The listing builds one solid part. Answer for the finished solid, in the listing's coordinates (mm). Face numbers are marked on the shaded views. A direction names the side the tool comes from. Round coordinates to 2 decimals unless told otherwise and drop trailing zeros. Order: outer loops, then holes, each group sorted by start corner. A loop starts at its lowest first (then second) coordinate and runs counter-clockwise, first axis right, second up. Notation, with made-up numbers: (-30, -8.5) - (-5, -8.5) arc R23 ccw to (-5, 13.5) - close; hole circle Ø2 at (28.25, 19.5). An arc over 180 degrees is marked (long way). One line per item, written item: value. Start each with the question number.
1. Section A-A, the plane z = 15.5 is taken. Give the vertices of the cut face in (x, y), then the cut area to 3 significant figures.
2. Flat-ended cylindrical pins translate along their axes: P1, Ø1, axis at x = -4, z = 14.5, coming from the +Y side; P2, Ø2, axis at x = -13, y = -5.5, coming from the -Z side; P3, Ø6, axis at x = -9.5, z = 15.5, coming from the -Y side; P4, Ø3.5, axis at y = -4, z = -7, coming from the +X side. Find the tip coordinate at first contact, or state that the pin passes through.
3. Straight lines are drawn through the part: line 1 (X direction, y = -5.75, z = 34.5); line 2 (X direction, y = -6.75, z = 40.5); line 3 (Z direction, x = -10, y = -0.55). For each, find the intervals that lie inside material, in ascending order.
4. Section C-C, the plane x = -1.5 is taken. Give the vertices of the cut face in (y, z), then the cut area to 4 significant figures.
5. Section D-D, the plane z = 8 is taken. Give the vertices of the cut face in (x, y).
6. Section B-B, the plane y = -10.5 is taken. Give the vertices of the cut face in (x, z), then the cut area to 4 significant figures.
7. A tool of negligible diameter and unlimited length cuts with its end or side. For the marked faces 1, 2, 3 and 4, from which of +Z, -Z, +X, -X, +Y, -Y can it reach the whole face along a straight path? Write none if from no direction.
from build123d import *

# Parameters (mm, degrees)
F0_W      = 8
F0_H      = 31
F1_DEPTH  = 20
F3_DEPTH  = 6.4
F4_R      = 2
F5_DEPTH  = 1.601
F9_W      = 4.8
F9_H      = 18
F10_DEPTH = 30
F12_DEPTH = 3
F13_R     = 2
F14_DEPTH = 1.801
F15_SIZE  = 0.5
F16_SIZE2 = 2
F16_SIZE  = 0.5
F17_SIZE  = 1


with BuildPart() as f1:
    # F0 (on Right) → F1 (new body)
    with BuildSketch(Plane.YZ):
        with Locations((-4, 15.5)):
            Rectangle(F0_W, F0_H)
    extrude(amount=-F1_DEPTH)

    # F2 (on face) → F3 (cut)
    with BuildSketch(Plane.XZ.offset(8)):
        Polygon((-6.45, 13.4504065444), (-6.45, 17.5495934556), (-10, 19.5991869112), (-13.55, 17.5495934556), (-13.55, 13.4504065444), (-10, 11.4008130888), align=None)
    extrude(amount=-F3_DEPTH, mode=Mode.SUBTRACT)

    # F4 (on face) → F5 (cut, through all)
    with BuildSketch(Plane.XZ.offset(1.6)):
        with Locations((-10, 15.5)):
            Circle(F4_R)
    extrude(amount=-F5_DEPTH, mode=Mode.SUBTRACT)

    # F9 (on 3pt) → F10 (join, symmetric)
    with BuildSketch(Plane.XY.offset(15.5)):
        with Locations((2.4, -4)):
            Rectangle(F9_W, F9_H)
    extrude(amount=F10_DEPTH, both=True)

    # F11 (on face) → F12 (cut)
    with BuildSketch(Plane(origin=(0, 0, 0), x_dir=(0, -1, 0), z_dir=(-1, 0, 0))):
        Polygon((6.0495934556, 41.55), (1.9504065444, 41.55), (-0.0991869112, 38), (1.9504065444, 34.45), (6.0495934556, 34.45), (8.0991869112, 38), align=None)
        Polygon((6.0495934556, -3.45), (1.9504065444, -3.45), (-0.0991869112, -7), (1.9504065444, -10.55), (6.0495934556, -10.55), (8.0991869112, -7), align=None)
    extrude(amount=-F12_DEPTH, mode=Mode.SUBTRACT)

    # F13 (on face) → F14 (cut, through all)
    with BuildSketch(Plane(origin=(3, 0, 0), x_dir=(0, -1, 0), z_dir=(-1, 0, 0))):
        with Locations((4, 38)):
            Circle(F13_R)
        with Locations((4, -7)):
            Circle(F13_R)
    extrude(amount=-F14_DEPTH, mode=Mode.SUBTRACT)

    # F15
    f15_edges = [f1.edges().sort_by_distance(p)[0] for p in [
        (-10, -8, 31),
        (-10, 0, 31),
        (-10, 0, 0),
        (-10, -8, 0),
        (-20, -8, 15.5),
        (-20, 0, 15.5),
    ]]
    chamfer(f15_edges, length=F15_SIZE)

    # F16
    f16_edges = [f1.edges().sort_by_distance(p)[0] for p in [
        (-20, -4, 31),
        (-20, -4, 0),
    ]]
    f16_side = f1.faces().sort_by_distance((-20, -4, 15.5))[0]
    chamfer(f16_edges, length=F16_SIZE, length2=F16_SIZE2, reference=f16_side)

    # F17
    f17_edges = [f1.edges().sort_by_distance(p)[0] for p in [
        (2.4, -13, 45.5),
        (2.4, 5, 45.5),
        (2.4, -13, -14.5),
        (2.4, 5, -14.5),
        (4.8, 5, 15.5),
        (4.8, -4, -14.5),
        (4.8, -13, 15.5),
        (0, -4, 45.5),
        (0, -4, -14.5),
    ]]
    chamfer(f17_edges, length=F17_SIZE)


solid = f1.part
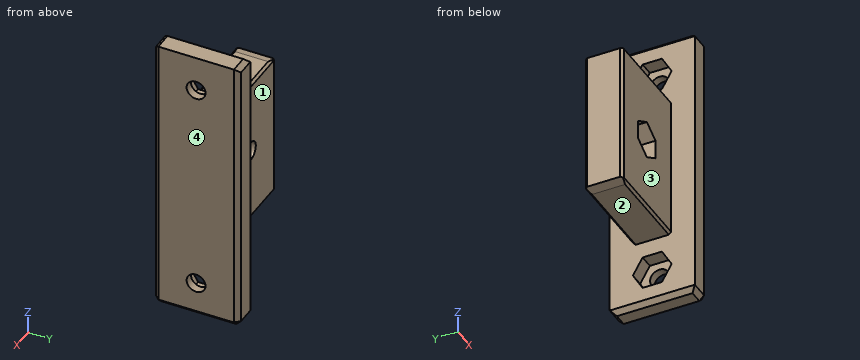
Answer list:
1. outline: (-20, -7.5) - (-19.5, -8) - (-13.55, -8) - (-13.55, -1.6) - (-12, -1.6) - (-12, 0) - (-19.5, 0) - (-20, -0.5) - close; (-8, -1.6) - (-6.45, -1.6) - (-6.45, -8) - (0, -8) - (0, -13) - (3.8, -13) - (4.8, -12) - (4.8, 4) - (3.8, 5) - (0, 5) - (0, 0) - (-8, 0) - close
1. area: 193 mm²
2. P1: stops at y = 0
2. P2: stops at z = 0
2. P3: stops at y = -1.6
2. P4: passes through
3. line 1: x = 3 to 4.8
3. line 2: x = 0 to 4.8
3. line 3: z = 0 to 13.5, 17.5 to 31
4. outline: (-8, 0.5) - (-7.5, 0) - (-0.5, 0) - (0, 0.5) - (0, 30.5) - (-0.5, 31) - (-7.5, 31) - (-8, 30.5) - close
4. area: 247.5 mm²
5. outline: (-20, -7.5) - (-19.5, -8) - (0, -8) - (0, -13) - (3.8, -13) - (4.8, -12) - (4.8, 4) - (3.8, 5) - (0, 5) - (0, 0) - (-19.5, 0) - (-20, -0.5) - close
6. outline: (0, -13.5) - (1, -14.5) - (3.8, -14.5) - (4.8, -13.5) - (4.8, 45.5) - (1, 45.5) - (0, 44.5) - close
6. area: 286.5 mm²
7. face 1: +Z, -Z, -X, +Y
7. face 2: -Z, -X, +Y, -Y
7. face 3: +Z, -Z, -X, -Y
7. face 4: +Z, -Z, +X, +Y, -Y
